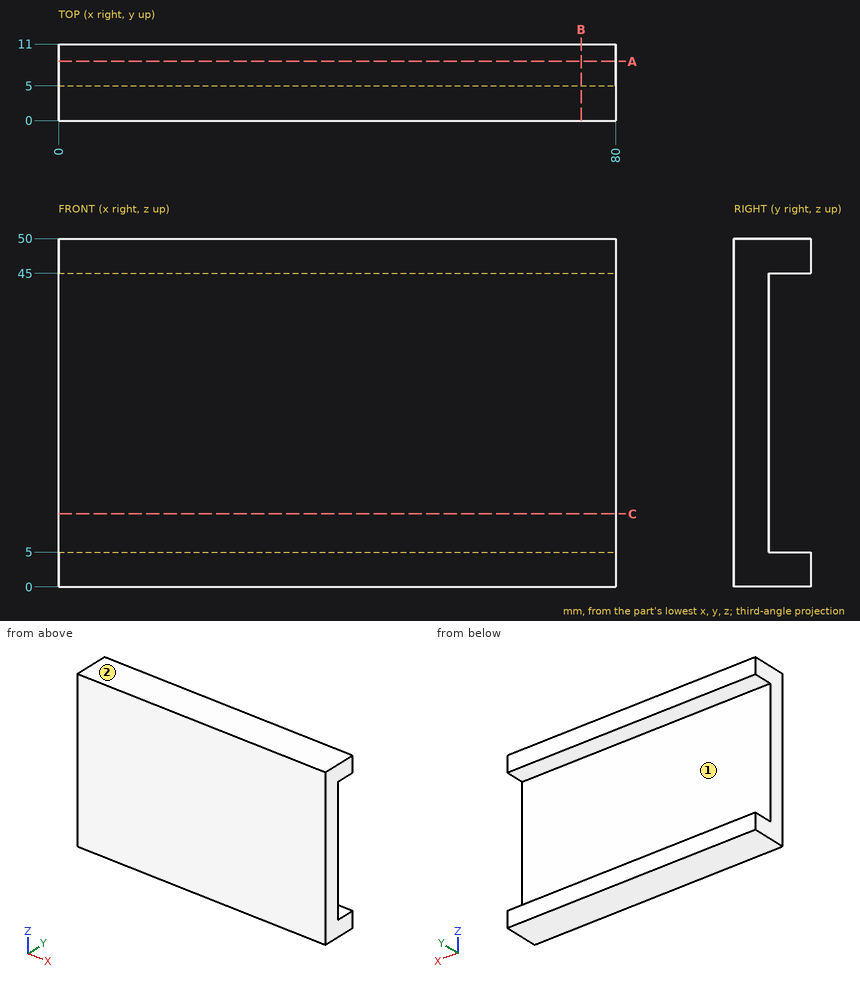
Input: dimensioned drawing with shaded views. Units: mm. Origin: part minimum x, y, z. A direction names the side the tool comes from. Round coordinates to 2 decimals unless told otherwise and drop trailing zeros. Order: outer loops, then holes, each group sorted by start corner. A loop starts at its lowest first (then second) coordinate and runs counter-clockwise, first axis right, second up. Notation, with made-up numbers: (-25.75, 49.5) -> (19.25, 49.5) arc R23 cw to (19.25, 76.5) -> close; hole circle Ø3 at (65.5, 76). An arc over 180 degrees is marked (long way). Put each result on its own line as item: value. Start each with the question number.
Q1. Section C-C on z = 10.5. Return the cut outline in (x, y), and give its area (3 significant figures).
Q2. First-contact query: pin 1 (20 mm diameter, centred on x = 45, z = 34.5, fed in from +Y); pin 2 (1 mm diameter, centred on x = 25.5, z = 15, fed in from -Y). Flat tips, straight axial feed; report the tip coordinate or a pass-through.
Q3. Reachability of the marked faces 1 and 2 from +Z, -Z, +X, -X, +Y, -Y: full face, straight path, thin tool, end or side. Return the list, or none.
Q4. Line query: probe 1 along Z at (x, y) = (26.5, 7.5); probe 2 along Y at (x, z) = (9, 13.5). Output: solid intervals per line, ascending.
Q5. Section B-B on x = 75. Return the cut outline in (y, z), and give its area (3 significant figures).
Q6. Section A-A on y = 8.5. Return the cut outline in (x, z).
Ans:
1. outline: (0, 0) -> (80, 0) -> (80, 5) -> (0, 5) -> close
1. area: 400 mm2
2. pin 1: stops at y = 5
2. pin 2: stops at y = 0
3. face 1: +X, -X, +Y
3. face 2: +Z, +X, -X, +Y, -Y
4. probe 1: z = 0 to 5, 45 to 50
4. probe 2: y = 0 to 5
5. outline: (0, 0) -> (11, 0) -> (11, 5) -> (5, 5) -> (5, 45) -> (11, 45) -> (11, 50) -> (0, 50) -> close
5. area: 310 mm2
6. outline: (0, 0) -> (80, 0) -> (80, 5) -> (0, 5) -> close; (0, 45) -> (80, 45) -> (80, 50) -> (0, 50) -> close
